Study the drawing (mm; zero at the part's minimum x, y, z) and answer. A direction names the side the tool comes from. Coordinates: 2 decimals unless noted, no trailing zeros. Order: outer loops, then holes, each group sorted by start corner. A loop starts at its lowest first (then second) coordinate and runs counter-clockwise, first axis right, second up.
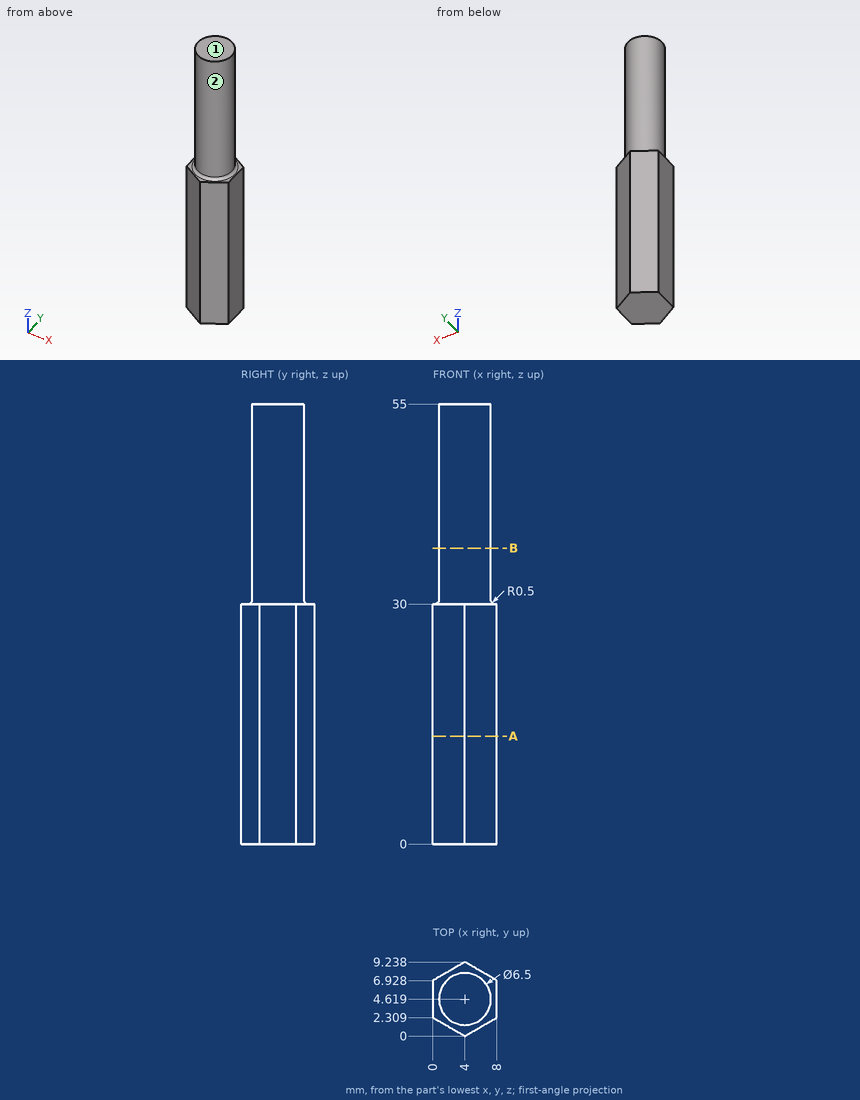
1) A cutting plane is placed at B-B, the plane z = 37. Determine the outline of the cut face in (x, y), and give its area (3 significant figures).
A:
outline: circle Ø6.5 at (4, 4.62)
area: 33.2 mm2
2) Straight lines are drawn through the part: line 1 (Z direction, x = 7, y = 6.75) (1 decimal); line 2 (X direction, y = 4.75, z = 46); line 3 (X direction, y = 2.25, z = 9) (1 decimal). For each, find the intervals that lie inside material, in ascending order.
A:
line 1: z = 0 to 30
line 2: x = 0.75 to 7.25
line 3: x = 0.1 to 7.9
3) Which of the six approach directions +Z, -Z, +X, -X, +Y, -Y give full straight-line access (tool end or side, diameter ignored) to the marked faces 1 and 2?
A:
face 1: +Z, +X, -X, +Y, -Y
face 2: +Z
4) A cutting plane is placed at A-A, the plane z = 13.5. Determine the outline of the cut face in (x, y), and give its area (3 significant figures).
A:
outline: (0, 2.31) - (4, 0) - (8, 2.31) - (8, 6.93) - (4, 9.24) - (0, 6.93) - close
area: 55.4 mm2
